Source: CAD feature listing. Evaluate the final solid. Frame: model axes, mm. Give positions to 0.01 mm unless a question says otherwise; leave off trailing zeros. Loops run counter-clockwise (first coordinate to the right, second up) from the corner with the lowest first, then second, coordinate; pieces in that order, holes last.
Autodesk Inventor part; units mm, degrees
ref_plane "YZ Plane" through (0, 0, 0) normal (1, 0, 0) x (0, 1, 0)
ref_plane "XZ Plane" through (0, 0, 0) normal (0, 1, 0) x (-1, 0, 0)
ref_plane "XY Plane" through (0, 0, 0) normal (0, 0, 1) x (1, 0, 0)
sketch "Sketch1" plane through (0, 0, 0) normal (0, 1, 0) x (-1, 0, 0)
  line L0 (0, 0) -> (0, -1219.2)
  line L1 (0, 0) -> (88.9, 0)
  line L2 (88.9, 0) -> (88.9, -1219.2)
  line L3 (88.9, -1219.2) -> (0, -1219.2)
  line L4 (0, 0) -> (0, 1219.2) construction
  line L5 (0, 1219.2) -> (1219.2, 1219.2) construction
  line L6 (0, 1219.2) -> (0, 3657.6) construction
  line L7 (0, 3657.6) -> (0, 4876.8) construction
  line L8 (0, 4876.8) -> (0, 6096) construction
  line L9 (0, -1219.2) -> (2438.4, -1219.2) construction
  line L10 (0, 6096) -> (2438.4, 6096) construction
  line L11 (2438.4, 6096) -> (2438.4, -1219.2) construction
  line L12 (0, 3657.6) -> (0, 3352.8) construction
  line L13 (0, 3352.8) -> (2438.4, 3352.8) construction
  line L14 (2438.4, 3352.8) -> (1219.2, 3352.8)
  line L15 (1219.2, 3352.8) -> (1219.2, 3263.9)
  line L16 (1219.2, 3263.9) -> (2438.4, 3263.9)
  line L17 (2438.4, 3263.9) -> (2438.4, 3352.8)
  line L18 (0, 6096) -> (862.1046, 6958.1046)
  line L19 (862.1046, 6958.1046) -> (924.9664, 6895.2428)
  line L20 (924.9664, 6895.2428) -> (62.8618, 6033.1382)
  line L21 (62.8618, 6033.1382) -> (0, 6096)
  line L22 (0, 4876.8) -> (1219.2, 4876.8) construction
  line L23 (1219.2, 4876.8) -> (2081.3046, 5738.9046)
  line L24 (1219.2, 1219.2) -> (2081.3046, 357.0954)
  line L25 (2081.3046, 357.0954) -> (2018.4428, 294.2336)
  line L26 (2018.4428, 294.2336) -> (1156.3382, 1156.3382)
  line L27 (1156.3382, 1156.3382) -> (1219.2, 1219.2)
  line L28 (2018.4428, 294.2336) -> (88.9, -1219.2)
  line L29 (2081.3046, 357.0954) -> (2144.1664, 419.9572)
  line L30 (2144.1664, 419.9572) -> (1282.0618, 1282.0618)
  line L31 (1282.0618, 1282.0618) -> (1219.2, 1219.2)
  line L32 (2438.4, 3352.8) -> (2438.4, 3441.7)
  line L33 (2438.4, 3441.7) -> (1219.2, 3441.7)
  line L34 (1219.2, 3441.7) -> (1219.2, 3352.8)
  line L35 (1156.3382, 4939.6618) -> (1282.0618, 4813.9382)
  line L36 (2018.4428, 5801.7664) -> (2144.1664, 5676.0428)
  line L37 (1282.0618, 4813.9382) -> (2144.1664, 5676.0428)
  line L38 (2018.4428, 5801.7664) -> (1156.3382, 4939.6618)
  line L39 (2018.4428, 5801.7664) -> (924.9664, 6895.2428)
  line L40 (62.8618, 6033.1382) -> (1156.3382, 4939.6618)
  line L41 (1233.6206, 4168.8855) -> (1267.6412, 4086.7527)
  line L42 (1263.7078, 2313.9849) -> (1230.0006, 2231.7229)
  arc A0 (862.1046, 6958.1046) -> (0, 6096) centre (431.0523, 6527.0523) ccw
  line L43 (1246.8542, 2272.8539) -> (2375.0183, 1810.583)
  line L44 (2391.8719, 1851.7139) -> (2358.1646, 1769.452)
  line L45 (2391.8719, 1851.7139) -> (1263.7078, 2313.9849)
  line L46 (1230.0006, 2231.7229) -> (2358.1646, 1769.452)
  line L47 (1230.0006, 2231.7229) -> (1219.2, 3263.9)
  line L48 (2144.1664, 419.9572) -> (2391.8719, 1851.7139)
  line L49 (2391.8719, 1851.7139) -> (2438.4, 3263.9)
  line L50 (1219.2, 3441.7) -> (1233.6206, 4168.8855)
  line L51 (1250.6309, 4127.8191) -> (2377.0248, 4594.3867)
  line L52 (2360.0145, 4635.4532) -> (2394.0351, 4553.3203)
  line L53 (2394.0351, 4553.3203) -> (1267.6412, 4086.7527)
  line L54 (2360.0145, 4635.4532) -> (1233.6206, 4168.8855)
  line L55 (2394.0351, 4553.3203) -> (2144.1664, 5676.0428)
  line L56 (2438.4, 3441.7) -> (2394.0351, 4553.3203)
  line L57 (2144.1664, 5676.0428) -> (2057.3895, 5656.7301)
  line L58 (2394.0351, 4553.3203) -> (2305.2058, 4549.7751)
  line L59 (2394.0351, 4553.3203) -> (2307.2582, 4534.0076)
  line L60 (2307.2582, 4534.0076) -> (2057.3895, 5656.7301)
  line L61 (2438.4, 3441.7) -> (2349.5707, 3438.1548)
  line L62 (2349.5707, 3438.1548) -> (2305.2058, 4549.7751)
  line L63 (1219.2, 3441.7) -> (1308.0825, 3439.9374)
  line L64 (1233.6206, 4168.8855) -> (1322.5031, 4167.1229)
  line L65 (1322.5031, 4167.1229) -> (1308.0825, 3439.9374)
  line L66 (2018.4428, 5801.7664) -> (1955.581, 5738.9046)
  line L67 (1955.581, 5738.9046) -> (862.1046, 6832.381)
  line L68 (924.9664, 6895.2428) -> (862.1046, 6832.381)
  line L69 (62.8618, 6033.1382) -> (125.7236, 6096)
  line L70 (62.8618, 6033.1382) -> (125.7236, 6096)
  line L71 (125.7236, 6096) -> (1219.2, 5002.5236)
  line L72 (1156.3382, 1156.3382) -> (0, 0)
  line L73 (0, 0) -> (62.8618, -62.8618)
  line L74 (1156.3382, 1156.3382) -> (1219.2, 1093.4764)
  line L75 (1219.2, 1093.4764) -> (62.8618, -62.8618)
  line L76 (2018.4428, 294.2336) -> (1963.5776, 364.1837)
  line L77 (88.9, -1219.2) -> (34.0348, -1149.2499)
  line L78 (34.0348, -1149.2499) -> (1963.5776, 364.1837)
  line L79 (2144.1664, 419.9572) -> (2056.5677, 435.1125)
  line L80 (2391.8719, 1851.7139) -> (2304.2732, 1866.8692)
  line L81 (2391.8719, 1851.7139) -> (2303.0201, 1854.6414)
  line L82 (2304.2732, 1866.8692) -> (2056.5677, 435.1125)
  line L83 (1230.0006, 2231.7229) -> (1318.8957, 2232.6531)
  line L84 (1219.2, 3263.9) -> (1308.0951, 3264.8302)
  line L85 (1308.0951, 3264.8302) -> (1318.8957, 2232.6531)
  line L86 (2438.4, 3263.9) -> (2349.5482, 3266.8275)
  line L87 (2349.5482, 3266.8275) -> (2303.0201, 1854.6414)
  line L88 (88.9, 0) -> (125.7236, 0)
  line L89 (1233.6206, 4168.8855) -> (1219.2, 4876.8)
  line L90 (1233.6206, 4168.8855) -> (1322.5022, 4170.6961)
  line L91 (1219.2, 4876.8) -> (1308.0816, 4878.6106)
  line L92 (1308.0816, 4878.6106) -> (1322.5022, 4170.6961)
  line L93 (1282.0618, 4813.9382) -> (1309.9674, 4786.0326)
  line L94 (1267.6412, 4086.7527) -> (1318.4756, 3964.0275)
  line L95 (2360.0145, 4635.4532) -> (2374.4273, 4641.4231)
  line L96 (1230.0006, 2231.7229) -> (1219.2, 1219.2)
  line L97 (1230.0006, 2231.7229) -> (1318.8955, 2230.7747)
  line L98 (1219.2, 1219.2) -> (1308.0949, 1218.2518)
  line L99 (1308.0949, 1218.2518) -> (1318.8955, 2230.7747)
  line L100 (1282.0618, 1282.0618) -> (1309.0636, 1309.0636)
  line L101 (1263.7078, 2313.9849) -> (1316.7428, 2438.4)
  line L102 (2358.1646, 1769.452) -> (2376.5379, 1763.082)
  point P0 (1770.957, 2057.4547)
  point P1 (1955.1236, 357.5528)
  point P2 (88.9, -1106.2164)
  point P3 (2292.1025, 1796.5213)
  point P4 (2067.2525, 496.8711)
  point P5 (1318.5187, 2195.4522)
  point P6 (1308.1049, 3263.9)
  point P7 (2349.4518, 3263.9)
  point P8 (2304.1085, 1887.6754)
  point P9 (2306.5112, 4517.0667)
  point P10 (2349.4292, 3441.7)
  point P11 (1308.1175, 3441.7)
  point P12 (2069.6708, 5601.5472)
  point P13 (2291.0394, 4606.8827)
  dimension "d0" = 1219.2
  dimension "d2" = 1219.2
  dimension "d3" = 1219.2
  dimension "d16" = 2438.4
  dimension "d17" = 1219.2
  dimension "d18" = 1219.2
  dimension "d20" = 2438.4
  dimension "d21" = 304.8
  dimension "d22" = 1219.2
  dimension "d23" = 88.9
  dimension "d24" = 1219.2
  dimension "d25" = 45
  dimension "d26" = 88.9
  dimension "d27" = 1219.2
  dimension "d28" = 1219.2
  dimension "d29" = 1219.2
  dimension "d31" = 1219.2
  dimension "d32" = 88.9
  dimension "d33" = 88.9
  dimension "d34" = 88.9
  dimension "d35" = 177.8
  dimension "d36" = 177.8
  dimension "d38" = 88.9
  dimension "d39" = 88.9
  dimension "d43" = 1219.2
  dimension "d44" = 88.9
  dimension "d45" = 1219.2
  dimension "d46" = 88.9
  dimension "d47" = 88.9
  dimension "d48" = 88.9
  dimension "d49" = 88.9
  dimension "d50" = 88.9
  dimension "d51" = 88.9
  dimension "d54" = 88.9
  dimension "d55" = 88.9
  dimension "d57" = 88.9
  dimension "d58" = 88.9
  dimension "d59" = 88.9
  dimension "d60" = 88.9
  dimension "d61" = 88.9
  dimension "d64" = 88.9
  dimension "d65" = 88.9
  dimension "d66" = 88.9
  dimension "d69" = 88.9
  dimension "d70" = 88.9
  dimension "d71" = 88.9
  dimension "d72" = 88.9
extrude "Extrusion1" add sketch "Sketch1" along normal blind 38.1 contours L52 L95 L55 | L95 L54 L60 L37 L55
properties part number "S_2x4x45.283"
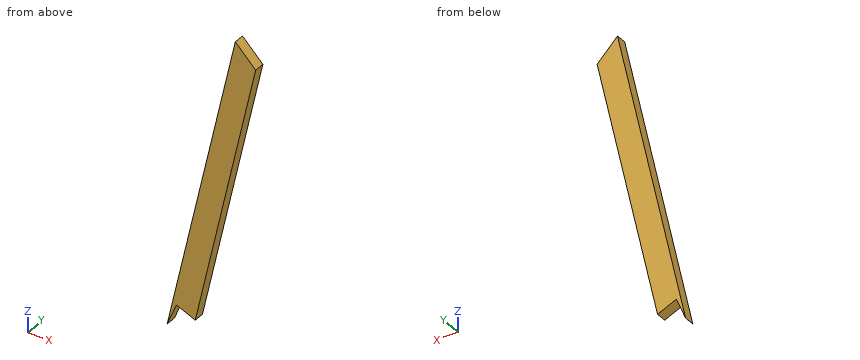
1) Cut plane A-A (y = 28). Return loops of the section in (x, z), and give its area (3 significant figures).
Checks:
outline: (-2394.04, 4553.32) - (-2360.01, 4635.45) - (-2291.04, 4606.88) - (-2069.67, 5601.55) - (-2144.17, 5676.04) - close
area: 93,100 mm2
2) Cut plane B-B (x = -2250). Return loops of the section in (y, z).
Checks:
outline: (0, 4791.28) - (38.1, 4791.28) - (38.1, 5200.51) - (0, 5200.51) - close
3) Contact query for flat-ended pins moving along their axis: P1, Ø1.5, axis at y = 13, z = 4836.5, coming from the +X side; P2, Ø5, axis at y = 6.5, z = 4847, coming from the -X side; P3, Ø5, axis at y = 15, z = 5438.5, coming from the -X side. Output: stop coordinate, or through.
Checks:
P1: stops at x = -2239.77
P2: stops at x = -2329.23
P3: stops at x = -2197.59
4) Ray query, probe 1 along X at (y, z) = (18.5, 5549); probe 2 along X at (y, z) = (28.5, 5534). Return the intervals inside material, ascending.
Checks:
probe 1: x = -2172.44 to -2081.37
probe 2: x = -2175.78 to -2084.7
5) Cut plane C-C (z = 4841.5). Return loops of the section in (x, y), and give its area (3 significant figures).
Checks:
outline: (-2329.9, 0) - (-2238.82, 0) - (-2238.82, 38.1) - (-2329.9, 38.1) - close
area: 3,470 mm2
